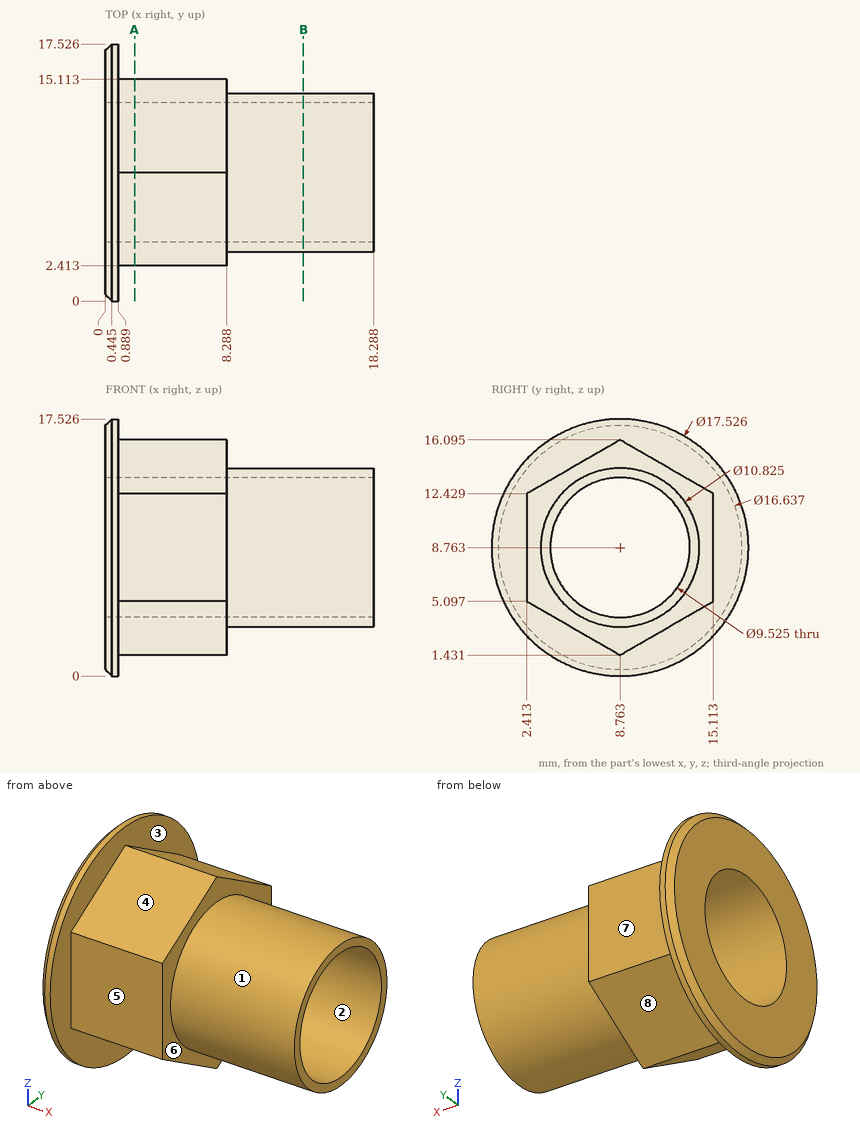
Geometry check sheet. Reference: drawing and pictorial views, mm from the part's lowest x, y, z. A direction names the side the tool comes from. Give positions to 0.01 mm unless a question says otherwise; leave off trailing zeros. Write each loop counter-clockwise with the first axis right and the second up, starting at its lowest first coordinate (ties: lowest second). Pieces come first, ordered by that corner, then holes. Notation, with made-up numbers: (-13, 77.5) - (-7, 77.5) arc R21 cw to (-7, 112.5) - close; hole circle Ø9 at (50.5, 64). An arc over 180 degrees is marked (long way). Use a Markdown table: item, result.
Q1. Thickness scan on L1, parallel to Y at x = 4, z = 9; L2, parallel to Y at x = 9.5, z = 12.25 (1 decimal); L3, parallel to Z at x = 5.5, y = 9.25 (1 decimal). Record the ranges inside material, lowest first. Write a range as [from, to].
Computed:
| item | result |
|---|---|
| L1 | y = [2.41, 4.01], [13.52, 15.11] |
| L2 | y = [4.6, 5.5], [12, 12.9] |
| L3 | z = [1.7, 4], [13.5, 15.8] |
Q2. Set-up check for the marked faces 5, 6, 7 and 8: record each of +Z, -Z, +X, -X, +Y, -Y from which the full face is reachable in a straight line by a thin tool's end or side.
Computed:
| item | result |
|---|---|
| face 5 | +Z, -Z, +X, -Y |
| face 6 | +X |
| face 7 | +Z, -Z, +X, +Y |
| face 8 | -Z, +X, +Y |
Q3. Draft check along Z on the marked faces 1, 2, 3 and 4. Enter one of: pulls with the +Z half, pulls with the -Z half, needs draft (parallel to the pull), parting line crosses it, or undercut.
Computed:
| item | result |
|---|---|
| face 1 | parting line crosses it |
| face 2 | undercut |
| face 3 | needs draft |
| face 4 | pulls with the +Z half |
Q4. Go/stop test with flat-tipped pins: P1, Ø2, axis at x = 4.5, z = 7, coming from the -Y side; P2, Ø8, axis at x = 4.5, y = 4.5, coming from the +Z side; P3, Ø10, axis at x = 14.5, z = 4.5, coming from the +Y side (1 decimal). Record where each tip stops, or that it passes through.
Computed:
| item | result |
|---|---|
| P1 | stops at y = 2.41 |
| P2 | stops at z = 17.15 |
| P3 | stops at y = 14.2 |
Q5. Section check A-A, the plane x = 2. Enter the section's corners in (y, z) (1 decimal).
Computed:
| item | result |
|---|---|
| outline | (2.4, 5.1) - (8.8, 1.4) - (15.1, 5.1) - (15.1, 12.4) - (8.8, 16.1) - (2.4, 12.4) - close; hole circle Ø9.5 at (8.8, 8.8) |
Q6. Section check B-B, the plane x = 13.5. Enter the section's corners in (y, z) (1 decimal).
Computed:
| item | result |
|---|---|
| outline | circle Ø10.8 at (8.8, 8.8); hole circle Ø9.5 at (8.8, 8.8) |
